from build123d import *

# Parameters (mm, degrees)
SKETCH_1_W              = 89
SKETCH_1_H              = 246
SKETCH_1_W_2            = 61
SKETCH_1_H_2            = 218
EXTRUDE_1_DEPTH         = 2
FILLET_1_R              = 5
FILLET_2_R              = 7
HOLE_WIZARD_1_OUTLINE_R = 3.3
HOLE_WIZARD_1_DEPTH     = 2


# Read off the part's stored shape, not the designer's step: 孔1
with BuildPart() as part:
    # 草图1 → 凸台-拉伸1 (new body)
    with BuildSketch(Plane.XY):
        Rectangle(SKETCH_1_W, SKETCH_1_H)
        Rectangle(SKETCH_1_W_2, SKETCH_1_H_2, mode=Mode.SUBTRACT)
    extrude(amount=EXTRUDE_1_DEPTH)

    # 圆角1
    fillet_1_edges = [part.edges().sort_by_distance(p)[0] for p in [
        (30.5, -109, 1),
        (30.5, 109, 1),
        (-30.5, 109, 1),
        (-30.5, -109, 1),
    ]]
    fillet(fillet_1_edges, radius=FILLET_1_R)

    # 圆角2
    fillet_2_edges = [part.edges().sort_by_distance(p)[0] for p in [
        (44.5, -123, 1),
        (-44.5, -123, 1),
        (-44.5, 123, 1),
        (44.5, 123, 1),
    ]]
    fillet(fillet_2_edges, radius=FILLET_2_R)

    # 孔1 outline → 孔1 (cut)
    with BuildSketch(Plane.XY):
        with Locations((36.5, 0)):
            Circle(HOLE_WIZARD_1_OUTLINE_R)
        with Locations((-36.5, 0)):
            Circle(HOLE_WIZARD_1_OUTLINE_R)
        with Locations((36.5, -115)):
            Circle(HOLE_WIZARD_1_OUTLINE_R)
        with Locations((-36.5, 115)):
            Circle(HOLE_WIZARD_1_OUTLINE_R)
        with Locations((-36.5, -115)):
            Circle(HOLE_WIZARD_1_OUTLINE_R)
        with Locations((36.5, 115)):
            Circle(HOLE_WIZARD_1_OUTLINE_R)
    extrude(amount=HOLE_WIZARD_1_DEPTH, mode=Mode.SUBTRACT)


solid = part.part
Read the model definition and answer for the solid it produces. Units are mm, in the model's axes. A direction names the side the tool comes from. Round coordinates to 2 decimals unless told otherwise and drop trailing zeros. Write each loop counter-clockwise with the first axis right and the second up, starting at its lowest first coordinate (ties: lowest second). Pieces come first, ordered by that corner, then holes. Notation, with made-up numbers: M 72,13 L 116,13 A21 cw 116,17 Z; hole C -31,60.25 d7. An arc over 180 degrees is marked long. Use a Markdown table: item, result.
1) The part is cut by section B-B (y = -85). Write down the section's boundary in (x, z).
Answers follow:
| item | result |
|---|---|
| outline | M -44.5,0 L -30.5,0 L -30.5,2 L -44.5,2 Z; M 30.5,0 L 44.5,0 L 44.5,2 L 30.5,2 Z |
2) A flat-ended cylindrical pin translates along its axis: pin 1 (6 mm diameter, centred on x = -36.5, y = 0, fed in from -Z). Find the tip coordinate at first contact, or state that the pin passes through.
Answers follow:
| item | result |
|---|---|
| pin 1 | passes through |
3) The part is cut by section A-A (x = 13). Write down the section's boundary in (y, z).
Answers follow:
| item | result |
|---|---|
| outline | M -123,0 L -109,0 L -109,2 L -123,2 Z; M 109,0 L 123,0 L 123,2 L 109,2 Z |
4) For a pull along X with two mould halves and no side action, classify faces 1 (the flat face through (33, 28, 0)), 2 (the cylindrical face through (42.4, -121, 1)), 3 (the cylindrical face through (29, -107.57, 1.01)), 4 (the cylindrical face through (38.02, -117.93, 0.99)) as pulls with the +X half, pulls with the -X half, needs draft (parallel to the pull), parting line crosses it, or undercut.
Answers follow:
| item | result |
|---|---|
| face 1 | needs draft |
| face 2 | pulls with the +X half |
| face 3 | undercut |
| face 4 | undercut |
5) Straight lines are drawn through the part: line 1 along Y through (x, z) = (-36.5, 1.3); line 2 along X through (y, z) = (-78.5, 1.8); line 3 along Y through (x, z) = (1.5, 0.5). For each, find the intervals that lie inside material, in ascending order. Write a range as [from, to].
Answers follow:
| item | result |
|---|---|
| line 1 | y = [-123, -118.3], [-111.7, -3.3], [3.3, 111.7], [118.3, 123] |
| line 2 | x = [-44.5, -30.5], [30.5, 44.5] |
| line 3 | y = [-123, -109], [109, 123] |
6) The part is cut by section C-C (y = 0). Write down the section's boundary in (x, z), plus the area to 3 significant figures.
Answers follow:
| item | result |
|---|---|
| outline | M -44.5,0 L -39.8,0 L -39.8,2 L -44.5,2 Z; M -33.2,0 L -30.5,0 L -30.5,2 L -33.2,2 Z; M 30.5,0 L 33.2,0 L 33.2,2 L 30.5,2 Z; M 39.8,0 L 44.5,0 L 44.5,2 L 39.8,2 Z |
| area | 29.6 mm2 |
7) A tool of negligible diameter and unlimited length cuts with its end or side. For faces 5 (the cylindrical face through (-42.5, 120.9, 1)), 6 (the cylindrical face through (-29, 107.57, 1.01)), from which of +Z, -Z, +X, -X, +Y, -Y can it reach the whole face along a straight path? Write none if from no direction.
Answers follow:
| item | result |
|---|---|
| face 5 | +Z, -Z, -X, +Y |
| face 6 | +Z, -Z |
